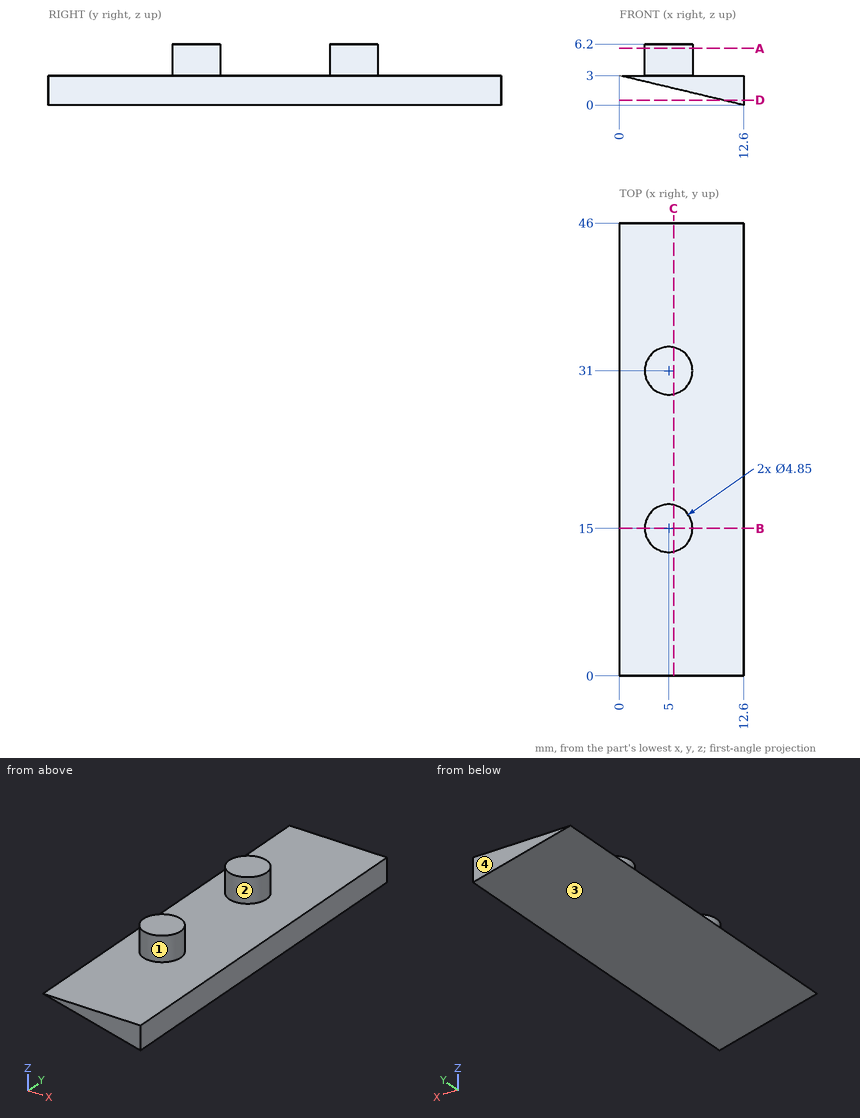
Job drawing, mm, ordinate dimensions from the low corner. One solid piece. Coordinates: 2 decimals unless noted, no trailing zeros. Write each loop counter-clockwise with the first axis right and the second up, starting at its lowest first coordinate (ties: lowest second). Pieces come first, ordered by that corner, then holes.
Item 1: Slice it at D-D (z = 0.5). Write the cut outline in (x, y), and give its area (3 significant figures).
Item 2: Probe line 1 (X direction, y = 15.5, z = 4.5); line 2 (Z direction, x = 11.5, y = 25); line 3 (Z direction, x = 2.75, y = 7). List the from-to ranges inside material, lowest first.
Item 3: Slice it at C-C (x = 5.5). Write the cut outline in (y, z).
Item 4: Slice it at A-A (z = 5.75). Write the cut outline in (x, y) (3 decimals), and give its area (3 significant figures).
Item 5: Pin check, flat tip, straight feed: pin 1 (2 mm diameter, centred on x = 10, y = 28.5, fed in from -Z). Stop position of the tip, or through.
Item 6: Mould opens along Y. For the marked faces 1, 2, 3 and 4 say: released by +Y, released by -Y, zero draft, split by the parting line, or undercut.
Item 7: Slice it at B-B (y = 15). Write the cut outline in (x, z) (3 decimals).
Results found:
1. outline: (10.5, 0) - (12.6, 0) - (12.6, 46) - (10.5, 46) - close
1. area: 96.6 mm2
2. line 1: x = 2.63 to 7.37
2. line 2: z = 0.26 to 3
2. line 3: z = 2.35 to 3
3. outline: (0, 1.69) - (46, 1.69) - (46, 3) - (33.37, 3) - (33.37, 6.2) - (28.63, 6.2) - (28.63, 3) - (17.37, 3) - (17.37, 6.2) - (12.63, 6.2) - (12.63, 3) - (0, 3) - close
4. outline: circle Ø4.85 at (5, 15); circle Ø4.85 at (5, 31)
4. area: 36.9 mm2
5. pin 1: stops at z = 0.38
6. face 1: undercut
6. face 2: undercut
6. face 3: zero draft
6. face 4: released by +Y
7. outline: (0, 3) - (12.6, 0) - (12.6, 3) - (7.425, 3) - (7.425, 6.2) - (2.575, 6.2) - (2.575, 3) - close
